Geometry check sheet. Reference: the model listing, model coordinates, mm. A direction names the side the tool comes from. Coordinates: 2 decimals unless noted, no trailing zeros. Write each loop counter-clockwise with the first axis right and the second up, starting at its lowest first coordinate (ties: lowest second). Pieces come first, ordered by that corner, then holes. Notation, with made-up numbers: M -31.75,-19 L 22.25,-19 A16 ccw 22.25,-10 Z; hole C -17,85 d2. An arc over 180 degrees is marked long. Answer as a JSON object with one key per item and string values. Group by question number.
Autodesk Inventor part; units mm, degrees
ref_plane "YZ Plane" through (0, 0, 0) normal (1, 0, 0) x (0, 1, 0)
ref_plane "XZ Plane" through (0, 0, 0) normal (0, 1, 0) x (-1, 0, 0)
ref_plane "XY Plane" through (0, 0, 0) normal (0, 0, 1) x (1, 0, 0)
sketch "Sketch1" plane through (0, 0, 0) normal (0, 1, 0) x (-1, 0, 0)
  line L0 (14.5, -14.5) -> (-14.5, -14.5)
  line L1 (-14.5, -14.5) -> (-14.5, 14.5)
  line L2 (-14.5, 14.5) -> (14.5, 14.5)
  line L3 (14.5, 14.5) -> (14.5, -14.5)
  dimension "d11" = 29
  dimension "d14" = 29
extrude "Extrusion1" add sketch "Sketch1" along normal blind 11
sketch "Sketch5" plane through (0, 11, 0) normal (0, 1, 0) x (1, 0, 0)
  line L0 (-1.6, 2.7) -> (1.6, 2.7)
  line L1 (1.6, 2.7) -> (1.6, -2.7)
  line L2 (1.6, -2.7) -> (-1.6, -2.7)
  line L3 (-1.6, -2.7) -> (-1.6, 2.7)
  point P0 (0, 0)
  dimension "d31" = 2.7
  dimension "d32" = 2.7
  dimension "d33" = 3.2
  dimension "d34" = 1.6
extrude "Extrusion4" cut sketch "Sketch5" against normal blind 6
equation "\"d14\" = d11"
properties part number "Motor_fit_check"
1) Go/stop test with a flat-tipped pin: pin 1 Ø5 at (x, z) = (-5.5, 11) entering from -Y. Record where the tip stops, or that it passes through.
2) Section check B-B (z = -2). Record the cut outline in (x, y).
3) Material ranges on probe 1 along X at (y, z) = (8, -2.25), recorded low to high. Write a range as [from, to].
4) Set-up check for faces 1 (the flat face through (0, 5, -14.5)), 2 (the flat face through (0, 5, 0)): record each of +Z, -Z, +X, -X, +Y, -Y from which the full face is reachable in a straight line by a thin tool's end or side.
5) Section check A-A (y = 8.5). Record the cut outline in (x, z).
6) Draft check along X on faces 3 (the flat face through (-14.5, 5, 0)), 4 (the flat face through (0, 0, 0)), 5 (the flat face through (0, 8, 2.7)). Enter one of: +X half, -X half, draft (parallel to the pull), parting line (faces both ways), or undercut.
Entries:
{
 "1": {"pin 1": "y = 0"},
 "2": {"outline": "M -14.5,0 L 14.5,0 L 14.5,11 L 1.6,11 L 1.6,5 L -1.6,5 L -1.6,11 L -14.5,11 Z"},
 "3": {"probe 1": "[-14.5, -1.6], [1.6, 14.5]"},
 "4": {"face 1": "-Z, +X, -X, +Y, -Y", "face 2": "+Y"},
 "5": {"outline": "M -14.5,-14.5 L 14.5,-14.5 L 14.5,14.5 L -14.5,14.5 Z; hole M -1.6,-2.7 L 1.6,-2.7 L 1.6,2.7 L -1.6,2.7 Z"},
 "6": {"face 3": "-X half", "face 4": "draft", "face 5": "undercut"}
}
